Build history of the part. All positions in model axes, mm. A direction names the side the tool comes from. Give positions to 0.01 mm unless a question says otherwise; leave off trailing zeros. Write each loop counter-clockwise with the first axis right and the second up, starting at its lowest first coordinate (ties: lowest second). Pieces come first, ordered by that corner, then holes. Notation, with made-up numbers: M -11.75,15 L 44.25,15 A12 ccw 44.25,25 Z; hole C 49.25,82.25 d10. An arc over 180 degrees is marked long. Return JSON: item names as keys, results as strings. Group by question number.
Q1. Band-saw the part on B-B, the plane z = -8. Give the cut face in (x, y).
Q2. Tool access for faces 1 (the flat face through (-3.9, -32, -15.2)), 2 (the flat face through (-18.818, -16, 4)): list every direction of +Z, -Z, +X, -X, +Y, -Y with a clear straight run to the whole face (end or side of a thin tool).
Q3. Pull direction X, two halves, no side cores. Call faces 3 (the cylindrical face through (-4.37, -13.52, -15.37)), 4 (the flat face through (-19.818, -16, 4)), 5 (the flat face through (-3.9, 0, -15.2)): +X half, -X half, draft (parallel to the pull), parting line (faces both ways), or undercut.
Q4. Wall check: probe 1 along X at (y, z) = (-5.5, -10); probe 2 along Z at (x, y) = (11.55, -16); probe 3 along X at (y, z) = (-16, -15.05). Give the ranges that are in metal, low to high.
Q5. Band-saw the part on D-D, the plane x = -4.5. Give the cut face in (y, z).
Q6. Flat gauge pins, fed straight in: pin 1 Ø15 at (x, y) = (-6, -24) entering from +Z; pin 2 Ø6 at (x, y) = (-3.82, -16) entering from -Z. Where does each tip first touch, or does it go through?
Q7. Band-saw the part on C-C, the plane y = -25.5. Give the cut face in (x, z).
Q8. Band-saw the part on A-A, the plane y = -16. Give the cut face in (x, z), then the cut area to 3 significant figures.
from build123d import *

# Parameters (mm, degrees)
F1_DEPTH = 32
F2_R     = 2.54
F3_DEPTH = 76.2
F4_R     = 2.54
F5_DEPTH = 25.4


with BuildPart() as f1:
    # F0 (on Front) → F1 (new body)
    with BuildSketch(Plane.XZ):
        Polygon((-18.817659, 16.140222), (-19.817659, 16.140222), (-19.817659, -15.859778), (12.182341, -15.859778), (12.182341, 16.140222), (11.182341, 16.140222), (11.182341, -14.859778), (-18.817659, -14.859778), align=None)
    extrude(amount=F1_DEPTH)

    # F2 (on face) → F3 (cut)
    with BuildSketch(Plane(origin=(-19.817659, 0, 0), x_dir=(0, -1, 0), z_dir=(-1, 0, 0))):
        with Locations((16, 0.140222)):
            Circle(F2_R)
    extrude(amount=-F3_DEPTH, mode=Mode.SUBTRACT)

    # F4 (on face) → F5 (cut)
    with BuildSketch(Plane(origin=(0, 0, -15.859778), x_dir=(1, 0, 0), z_dir=(0, 0, -1))):
        with Locations((-3.817659, 16)):
            Circle(F4_R)
    extrude(amount=-F5_DEPTH, mode=Mode.SUBTRACT)


solid = f1.part
From the geometry:
{
 "1": {"outline": "M -19.82,-32 L -18.82,-32 L -18.82,0 L -19.82,0 Z; M 11.18,-32 L 12.18,-32 L 12.18,0 L 11.18,0 Z"},
 "2": {"face 1": "+Z, -Z, +X, -X, -Y", "face 2": "+Z, +Y, -Y"},
 "3": {"face 3": "undercut", "face 4": "-X half", "face 5": "draft"},
 "4": {"probe 1": "x = -19.82 to -18.82, 11.18 to 12.18", "probe 2": "z = -15.86 to -2.4, 2.68 to 16.14", "probe 3": "x = -19.82 to -6.36, -1.28 to 12.18"},
 "5": {"outline": "M -32,-15.86 L -18.45,-15.86 L -18.45,-14.86 L -32,-14.86 Z; M -13.55,-15.86 L 0,-15.86 L 0,-14.86 L -13.55,-14.86 Z"},
 "6": {"pin 1": "stops at z = -14.86", "pin 2": "stops at z = -15.86"},
 "7": {"outline": "M -19.82,-15.86 L 12.18,-15.86 L 12.18,16.14 L 11.18,16.14 L 11.18,-14.86 L -18.82,-14.86 L -18.82,16.14 L -19.82,16.14 Z"},
 "8": {"outline": "M -19.82,-15.86 L -6.36,-15.86 L -6.36,-14.86 L -18.82,-14.86 L -18.82,-2.4 L -19.82,-2.4 Z; M -19.82,2.68 L -18.82,2.68 L -18.82,16.14 L -19.82,16.14 Z; M -1.28,-15.86 L 12.18,-15.86 L 12.18,-2.4 L 11.18,-2.4 L 11.18,-14.86 L -1.28,-14.86 Z; M 11.18,2.68 L 12.18,2.68 L 12.18,16.14 L 11.18,16.14 Z", "area": "78.8 mm^2"}
}
